Autodesk Fusion 360 part; units mm, degrees
sketch "Sketch1" plane through (0, 0, 0) normal (0, 0, 1) x (1, 0, 0)
  line L0 (0, 47.8) -> (49.4, 47.8)
  line L1 (49.4, 47.8) -> (49.4, 0)
  line L2 (49.4, 0) -> (0, 0)
  line L3 (0, 0) -> (0, 47.8)
  line L4 (10, 47.8) -> (10, 50.8)
  line L5 (10, 50.8) -> (39.4, 50.8)
  line L6 (39.4, 50.8) -> (39.4, 47.8)
  line L7 (49.4, 45.8) -> (53, 45.8)
  line L8 (53, 45.8) -> (53, 30.8)
  line L9 (53, 30.8) -> (49.4, 30.8)
  line L10 (49.4, 15) -> (53, 15)
  line L11 (53, 15) -> (53, 5)
  line L12 (53, 5) -> (49.4, 5)
  line L13 (0, 41.8) -> (-3, 41.8)
  line L14 (-3, 41.8) -> (-3, 32.8)
  line L15 (-3, 32.8) -> (0, 32.8)
  line L16 (2, 0) -> (2, -3)
  line L17 (2, -3) -> (15, -3)
  line L18 (15, -3) -> (15, 0)
  line L19 (0, 5) -> (-3, 5)
  line L20 (-3, 5) -> (-3, 15)
  line L21 (-3, 15) -> (0, 15)
  line L22 (8.5, 36.8) -> (8.5, 26.8)
  line L23 (8.5, 26.8) -> (8, 26.8)
  line L24 (8, 26.8) -> (8, 40.8)
  line L25 (8, 40.8) -> (17, 40.8)
  line L26 (17, 40.8) -> (17, 26.8)
  line L27 (17, 26.8) -> (16.5, 26.8)
  line L28 (16.5, 26.8) -> (16.5, 36.8)
  line L29 (16.5, 36.8) -> (8.5, 36.8)
  line L30 (9.5, 39.8) -> (9.5, 37.8)
  line L31 (9.5, 37.8) -> (15.5, 37.8)
  line L32 (15.5, 37.8) -> (15.5, 39.8)
  line L33 (15.5, 39.8) -> (9.5, 39.8)
  line L34 (8.5, 36.8) -> (8.5, 40.4566)
  line L35 (8.5, 40.4566) -> (16.5, 40.4566)
  line L36 (16.5, 40.4566) -> (16.5, 36.8)
  line L37 (8.5, 26.8) -> (16.5, 26.8)
  line L38 (33.9, 39.8) -> (33.9, 37.8)
  line L39 (32.9, 36.8) -> (32.9, 40.4566)
  line L40 (32.9, 26.8) -> (32.4, 26.8)
  line L41 (32.4, 26.8) -> (32.4, 40.8)
  line L42 (40.9, 26.8) -> (40.9, 36.8)
  line L43 (40.9, 36.8) -> (32.9, 36.8)
  line L44 (32.4, 40.8) -> (41.4, 40.8)
  line L45 (40.9, 40.4566) -> (40.9, 36.8)
  line L46 (32.9, 36.8) -> (32.9, 26.8)
  line L47 (41.4, 40.8) -> (41.4, 26.8)
  line L48 (32.9, 40.4566) -> (40.9, 40.4566)
  line L49 (41.4, 26.8) -> (40.9, 26.8)
  line L50 (32.9, 26.8) -> (40.9, 26.8)
  line L51 (33.9, 37.8) -> (39.9, 37.8)
  line L52 (39.9, 37.8) -> (39.9, 39.8)
  line L53 (39.9, 39.8) -> (33.9, 39.8)
  line L54 (16.5, 11) -> (16.5, 7.3434)
  line L55 (40.9, 11) -> (40.9, 7.3434)
  line L56 (39.9, 8) -> (39.9, 10)
  line L57 (16.5, 21) -> (17, 21)
  line L58 (41.4, 21) -> (41.4, 7)
  line L59 (15.5, 10) -> (9.5, 10)
  line L60 (32.9, 11) -> (40.9, 11)
  line L61 (16.5, 11) -> (16.5, 21)
  line L62 (15.5, 8) -> (15.5, 10)
  line L63 (40.9, 21) -> (41.4, 21)
  line L64 (9.5, 8) -> (15.5, 8)
  line L65 (40.9, 11) -> (40.9, 21)
  line L66 (16.5, 7.3434) -> (8.5, 7.3434)
  line L67 (40.9, 21) -> (32.9, 21)
  line L68 (32.4, 21) -> (32.9, 21)
  line L69 (9.5, 10) -> (9.5, 8)
  line L70 (41.4, 7) -> (32.4, 7)
  line L71 (33.9, 8) -> (39.9, 8)
  line L72 (40.9, 7.3434) -> (32.9, 7.3434)
  line L73 (39.9, 10) -> (33.9, 10)
  line L74 (32.9, 7.3434) -> (32.9, 11)
  line L75 (33.9, 10) -> (33.9, 8)
  line L76 (17, 21) -> (17, 7)
  line L77 (8, 7) -> (8, 21)
  line L78 (32.4, 7) -> (32.4, 21)
  line L79 (8.5, 7.3434) -> (8.5, 11)
  line L80 (16.5, 21) -> (8.5, 21)
  line L81 (8.5, 21) -> (8.5, 11)
  line L82 (17, 7) -> (8, 7)
  line L83 (32.9, 21) -> (32.9, 11)
  line L84 (8, 21) -> (8.5, 21)
  line L85 (8.5, 11) -> (16.5, 11)
  point P0 (24.7, 23.9)
  dimension "d1" = 49.4
  dimension "d2" = 47.8
  dimension "d3" = 2
  dimension "d4" = 15
  dimension "d5" = 3
  dimension "d6" = 5
  dimension "d7" = 10
  dimension "d8" = 3
  dimension "d9" = 6
  dimension "d10" = 15
  dimension "d11" = 3
  dimension "d12" = 10
  dimension "d13" = 10
  dimension "d14" = 3
  dimension "d15" = 2
  dimension "d16" = 15
  dimension "d17" = 5
  dimension "d18" = 10
  dimension "d19" = 0.5
  dimension "d20" = 0.5
  dimension "d21" = 10
  dimension "d23" = 1
  dimension "d24" = 1
  dimension "d26" = 2
  dimension "d27" = 1
  dimension "d28" = 1
  dimension "d29" = 7
  dimension "d30" = 8
  dimension "d31" = 24.7
  dimension "d32" = 23.9
  dimension "d33" = 8
  dimension "d34" = 9
  dimension "d37" = 24.4
  dimension "d38" = 0
  dimension "d40" = 360
extrude "Extrude1" add sketch "Sketch1" along normal blind 2 contours L0 L1 L2 L3 | L0 L4 L5 L6 | L3 L13 L14 L15 | L3 L19 L20 L21 | L1 L7 L8 L9 | L1 L10 L11 L12 | L2 L16 L17 L18 | L22 L28 L29 L37 | L29 L34 L35 L36 | L30 L31 L32 L33 | L38 L51 L52 L53 | L39 L43 L45 L48 | L42 L43 L46 L50 | L61 L80 L81 L85 | L54 L66 L79 L85 | L55 L60 L72 L74 | L60 L65 L67 L83 | L56 L71 L73 L75 | L59 L62 L64 L69
extrude "Extrude2" cut sketch "Sketch1" against normal blind 0.8 from surface at 2 contours L22 L28 L29 L37 | L42 L43 L46 L50 | L61 L80 L81 L85 | L60 L65 L67 L83
extrude "Extrude3" add sketch "Sketch1" along normal blind 1.5 from surface at 2 contours L30 L31 L32 L33 | L38 L51 L52 L53 | L56 L71 L73 L75 | L59 L62 L64 L69
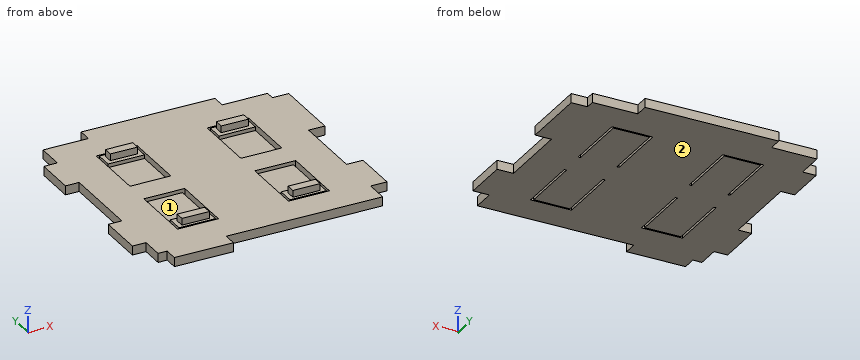
Part model, mm, in its own coordinate system. Face numbers are marked on the shaded views. Give positions to 0.01 mm unless a question says otherwise; leave off trailing zeros. Order: outer loops, then holes, each group sorted by start corner. A loop starts at its lowest first (then second) coordinate and runs counter-clockwise, first axis right, second up. Notation, with made-up numbers: M 40.25,76 L 67.25,76 A10 ccw 67.25,82 Z; hole C 8.5,84 d6. An arc over 180 degrees is marked long. Use a Markdown table: item, result. Add a question column.
(1) Saw through at B-B, the plane z = 2.85. Give the cut face in (x, y), and give its area (3 significant figures).
(2) Mould opens along Y. For the marked faces 1 and 2 say: +Y half, -Y half, draft (parallel to the pull), parting line (faces both ways), or undercut.
(3) Saw through at C-C, the plane x = 38. Give the cut face in (y, z).
(4) Probe line 1 along Y through (x, z) = (35, 1.5); line 2 along Y through (x, z) = (9, 1.9); line 3 along X through (y, z) = (28, 1.3). List the from-to ranges inside material, lowest first. Write a range as [from, to].
(5) Saw through at A-A, the plane y = 20. Give the cut face in (x, z), and give its area (3 significant figures).
(6) Saw through at D-D, the plane y = 38.5. Give the cut face in (x, z), and give its area (3 significant figures).
(7) Drop flat-ended pins along their axis: P1, Ø1.6, axis at x = 44, z = 1, coming from the +Y side; P2, Ø2, axis at y = 20, z = 1, coming from the -X side; P3, Ø1.6, axis at x = -1, z = 1, coming from the -Y side; P4, Ø1.6, axis at y = 38.5, z = 2.5, coming from the -X side. Give the stop position or say it passes through.
Answer key:
| question | item | result |
|---|---|---|
| 1 | outline | M 9.5,8 L 15.5,8 L 15.5,10 L 9.5,10 Z; M 9.5,37.8 L 15.5,37.8 L 15.5,39.8 L 9.5,39.8 Z; M 33.9,8 L 39.9,8 L 39.9,10 L 33.9,10 Z; M 33.9,37.8 L 39.9,37.8 L 39.9,39.8 L 33.9,39.8 Z |
| 1 | area | 48.0 mm^2 |
| 2 | face 1 | undercut |
| 2 | face 2 | draft |
| 3 | outline | M 0,0 L 7,0 L 7,2 L 0,2 Z; M 7.34,0 L 40.46,0 L 40.46,2 L 39.8,2 L 39.8,3.5 L 37.8,3.5 L 37.8,2 L 36.8,2 L 36.8,1.2 L 26.8,1.2 L 26.8,2 L 21,2 L 21,1.2 L 11,1.2 L 11,2 L 10,2 L 10,3.5 L 8,3.5 L 8,2 L 7.34,2 Z; M 40.8,0 L 50.8,0 L 50.8,2 L 40.8,2 Z |
| 4 | line 1 | [0, 7], [7.34, 11], [21, 26.8], [36.8, 40.46], [40.8, 50.8] |
| 4 | line 2 | [-3, 7], [7.34, 11], [21, 26.8], [36.8, 40.46], [40.8, 47.8] |
| 4 | line 3 | [0, 8], [17, 32.4], [41.4, 49.4] |
| 5 | outline | M 0,0 L 8,0 L 8,2 L 0,2 Z; M 8.5,0 L 16.5,0 L 16.5,1.2 L 8.5,1.2 Z; M 17,0 L 32.4,0 L 32.4,2 L 17,2 Z; M 32.9,0 L 40.9,0 L 40.9,1.2 L 32.9,1.2 Z; M 41.4,0 L 49.4,0 L 49.4,2 L 41.4,2 Z |
| 5 | area | 82.0 mm^2 |
| 6 | outline | M -3,0 L 8,0 L 8,2 L -3,2 Z; M 8.5,0 L 16.5,0 L 16.5,2 L 15.5,2 L 15.5,3.5 L 9.5,3.5 L 9.5,2 L 8.5,2 Z; M 17,0 L 32.4,0 L 32.4,2 L 17,2 Z; M 32.9,0 L 40.9,0 L 40.9,2 L 39.9,2 L 39.9,3.5 L 33.9,3.5 L 33.9,2 L 32.9,2 Z; M 41.4,0 L 53,0 L 53,2 L 41.4,2 Z |
| 6 | area | 126 mm^2 |
| 7 | P1 | y = 47.8 |
| 7 | P2 | x = 0 |
| 7 | P3 | y = 5 |
| 7 | P4 | x = -3 |
